```python
from build123d import *

# Parameters (mm, degrees)
F1_DEPTH = 990
F2_R     = 4.6
F3_R     = 14
F5_D     = 25
F7_D     = 25
F9_D     = 25
F11_D    = 25


with BuildPart() as f1:
    # F0 (on Top) → F1 (new body)
    with BuildSketch(Plane.XY):
        Polygon((0, 125), (0, 0), (125, 0), (125, 12), (12, 12), (12, 125), align=None)
    extrude(amount=F1_DEPTH)

    # F2
    f2_edges = [f1.edges().sort_by_distance(p)[0] for p in [
        (12, 125, 495),
        (125, 12, 495),
    ]]
    fillet(f2_edges, radius=F2_R)

    # F3
    f3_edges = [f1.edges().sort_by_distance(p)[0] for p in [
        (12, 12, 495),
    ]]
    fillet(f3_edges, radius=F3_R)

    # F5 (through all)
    with Locations(Plane(origin=(0, 0, 0), x_dir=(0, -1, 0), z_dir=(-1, 0, 0))):
        with Locations((-57.285432, 908.028543), (-59.564956, 459.623039), (-59.564956, 547.018707), (-59.564956, 624.141753), (-59.564956, 683.498025), (-59.564956, 748.724401), (-57.285432, 827.314973)):
            Hole(F5_D / 2)

    # F7 (through all)
    with Locations(Plane(origin=(0, 0, 0), x_dir=(0, -1, 0), z_dir=(-1, 0, 0))):
        with Locations((-72.530732, 202.228412)):
            Hole(F7_D / 2)

    # F9 (through all)
    with Locations(Plane.YZ.offset(12)):
        with Locations((65.758131, 26.347905)):
            Hole(F9_D / 2)

    # F11 (through all)
    with Locations(Plane.YZ.offset(12)):
        with Locations((65.283261, 98.539941)):
            Hole(F11_D / 2)


solid = f1.part
```
The model under review builds one solid part; all positions refer to its coordinate system, in mm. A direction names the side the tool comes from. Give positions to 0.01 mm unless a question says otherwise; leave off trailing zeros. Loops run counter-clockwise (first coordinate to the right, second up) from the corner with the lowest first, then second, coordinate; pieces in that order, holes last. Notation, with made-up numbers: (70, 34) -> (96, 34) arc R23 ccw to (96, 62) -> close; hole circle Ø2 at (65, 47). An arc over 180 degrees is marked (long way). Use CSV: the item, a comma, the result in double quotes.
1. Machinability: for faces 1 (the face through (12, 73, 488)), 2 (the face through (6.084, 65.333, 672.408)), which of the approach directions +Z, -Z, +X, -X, +Y, -Y give a long, thin tool a straight path to every point of the face, cutting with its end or side? Answer none if there is none.
Result:
face 1,"+Z, -Z, +X, +Y"
face 2,"+X, -X"
2. For P1, Ø12, axis at x = 59.5, z = 684, coming from the +Y side, flat-tipped, find the tip position at first contact; note if it passes through.
Result:
P1,"stops at y = 12"
3. Consider section B-B, the plane y = 101. Write out the cut boundary in (x, z).
Result:
outline,"(0, 0) -> (12, 0) -> (12, 990) -> (0, 990) -> close"
4. To check wall thickness, follow probe 1 along X at (y, z) = (56, 46.5); probe 2 along Y at (x, z) = (10, 468). State the ranges of each line that lie inside material, in increasing order. Write a range as from..to.
Result:
probe 1,"x = 0..12"
probe 2,"y = 0..50.29, 68.84..124.19"
5. Consider section A-A, the plane z = 232.5. Write out the cut boundary in (x, y), then the cut area to 3 significant figures.
Result:
outline,"(0, 0) -> (125, 0) -> (125, 7.4) arc R4.6 ccw to (120.4, 12) -> (26, 12) arc R14 cw to (12, 26) -> (12, 120.4) arc R4.6 ccw to (7.4, 125) -> (0, 125) -> close"
area,"2,890 mm²"
6. The part is to be moulded in two halves that separate along Z. For faces 3 (the face through (11, 40, 0)), 4 (the face through (11, 40, 990)), 5 (the face through (6.084, 57.938, 559.412)), 6 (the face through (74, 12, 488)), say which applies: +Z half, -Z half, draft (parallel to the pull), parting line (faces both ways), or undercut.
Result:
face 3,"-Z half"
face 4,"+Z half"
face 5,"undercut"
face 6,"draft"
